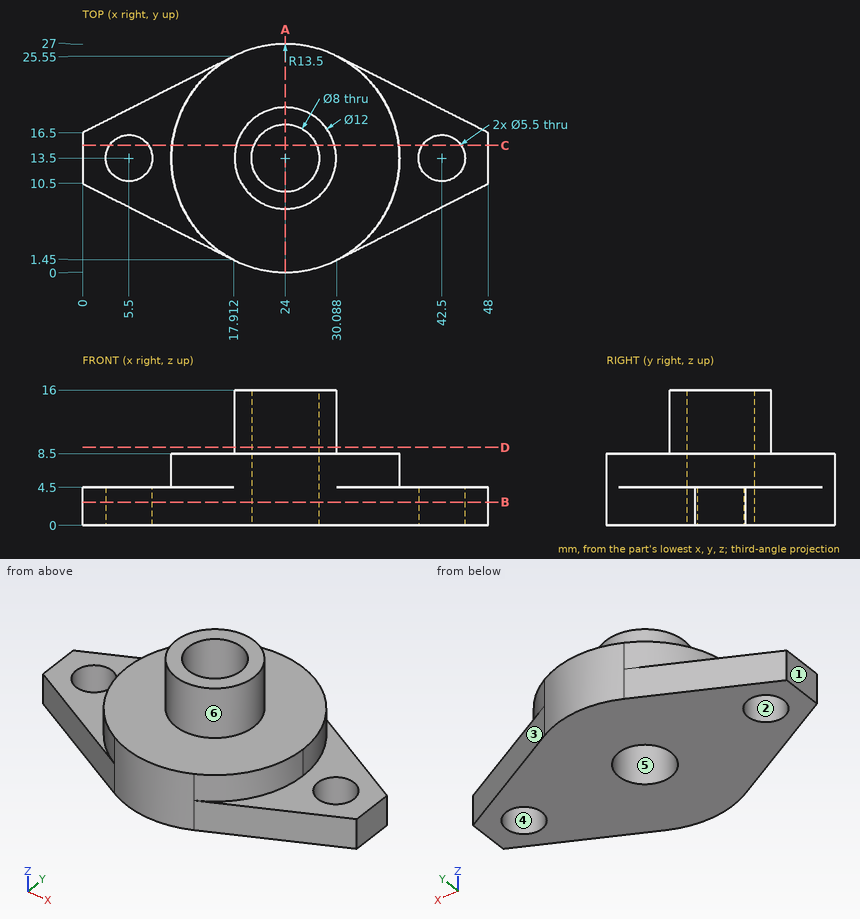
Can you work these out from the drawing? Everything is in mm from the part's minimum corner. A direction names the side the tool comes from. Round coordinates to 2 decimals unless told otherwise and drop trailing zeros. Loops run counter-clockwise (first coordinate to the right, second up) from the corner with the lowest first, then second, coordinate; pieces in that order, holes last.
1. We'd pull the mould along Y, two halves only. Please class the marked faces 1, 2, 3 and 4: +Y half, -Y half, draft (parallel to the pull), parting line (faces both ways), or undercut.
Answer list:
face 1: draft
face 2: undercut
face 3: +Y half
face 4: undercut
2. For P1, Ø1.5, axis at x = 25, y = 21.5, coming from the +Z side; P2, Ø3, axis at x = 40.5, y = 21, coming from the +Z side; P3, Ø1, axis at x = 8.5, z = 6, coming from the -Y side; P4, Ø2, axis at x = 14.5, z = 6.5, coming from the +Y side, each with a flat end and sliding along its axis, tell me the tip position at first contact or that it passes through.
Answer list:
P1: stops at z = 8.5
P2: stops at z = 4.5
P3: passes through
P4: stops at y = 23.99
3. If we section it at B-B on z = 2.75: Write out the boundary of the cut face in (x, y).
Answer list:
outline: (0, 10.5) - (17.91, 1.45) arc R13.5 ccw to (30.09, 1.45) - (48, 10.5) - (48, 16.5) - (30.09, 25.55) arc R13.5 ccw to (17.91, 25.55) - (0, 16.5) - close; hole circle Ø5.5 at (5.5, 13.5); hole circle Ø8 at (24, 13.5); hole circle Ø5.5 at (42.5, 13.5)
4. If we section it at D-D on z = 9.25: Write out the boundary of the cut face in (x, y).
Answer list:
outline: circle Ø12 at (24, 13.5); hole circle Ø8 at (24, 13.5)
5. If I drill on line 1 along X through (y, z) = (13.5, 2.65); line 2 along X through (y, z) = (13.5, 5.5); line 3 along Y through (x, z) = (24, 7), over which ranges is the centre line in solid material (lowest first)?
Answer list:
line 1: x = 0 to 2.75, 8.25 to 20, 28 to 39.75, 45.25 to 48
line 2: x = 10.5 to 20, 28 to 37.5
line 3: y = 0 to 9.5, 17.5 to 27
6. If we section it at A-A on x = 24: Write out the boundary of the cut face in (y, z).
Answer list:
outline: (0, 0) - (9.5, 0) - (9.5, 16) - (7.5, 16) - (7.5, 8.5) - (0, 8.5) - close; (17.5, 0) - (27, 0) - (27, 8.5) - (19.5, 8.5) - (19.5, 16) - (17.5, 16) - close
7. If we section it at C-C on y = 15: Write out the boundary of the cut face in (x, z) (1 decimal).
Answer list:
outline: (0, 0) - (3.2, 0) - (3.2, 4.5) - (0, 4.5) - close; (7.8, 0) - (20.3, 0) - (20.3, 16) - (18.2, 16) - (18.2, 8.5) - (10.6, 8.5) - (10.6, 4.5) - (7.8, 4.5) - close; (27.7, 0) - (40.2, 0) - (40.2, 4.5) - (37.4, 4.5) - (37.4, 8.5) - (29.8, 8.5) - (29.8, 16) - (27.7, 16) - close; (44.8, 0) - (48, 0) - (48, 4.5) - (44.8, 4.5) - close
8. Which directions (+Z, -Z, +X, -X, +Y, -Y) give clear straight access to the entire face, cutting with the end or side of a thin tool? Please do the marked faces 5 and 6.
Answer list:
face 5: +Z, -Z
face 6: +Z
